The figure shows three views and two pictorial views of one solid part (mm, origin at its lowest corner). Answer the questions. A direction names the side the tool comes from. Coordinates: 2 decimals unless noted, no trailing zeros. Loops run counter-clockwise (first coordinate to the right, second up) from the corner with the lowest first, then second, coordinate; pieces in that order, holes last. Notation, with made-up numbers: M 53,39 L 86,39 A34 cw 86,71 Z; hole C -26,82.5 d5. An arc over 180 degrees is marked long. Return JSON: item names as keys, results as strings. Group by question number.
1. Given P1, Ø2, axis at x = 37, y = 4, coming from the -Z side, flat-ended and moving along its own axis, determine where the tip first touches the part or whether it passes through.
2. Straight lines are drawn through the part: L1, parallel to X at y = 3.15, z = 11; L2, parallel to X at y = 4.6, z = 5; L3, parallel to Z at x = 25, y = 1.6. For each, find the intervals that lie inside material, in ascending order. Write a range as from..to.
3. Which of the six approach directions +Z, -Z, +X, -X, +Y, -Y give full straight-line access (tool end or side, diameter ignored) to the marked faces 1 and 2?
4. Section C-C (y = 4.2) is taken. Write down the section's boundary in (x, z).
5. Section D-D (x = 10.75) is taken. Write down the section's boundary in (y, z), then the cut area to 3 significant figures.
6. Section A-A (x = 24) is taken. Write down the section's boundary in (y, z), then the cut area to 3 significant figures.
7. The mould has two halves that part along X. Classify the marked faces 3, 4 and 5: pulls with the +X half, pulls with the -X half, needs draft (parallel to the pull), parting line crosses it, or undercut.
8. Section B-B (z = 11) is taken. Write down the section's boundary in (x, y), then the cut area to 3 significant figures.
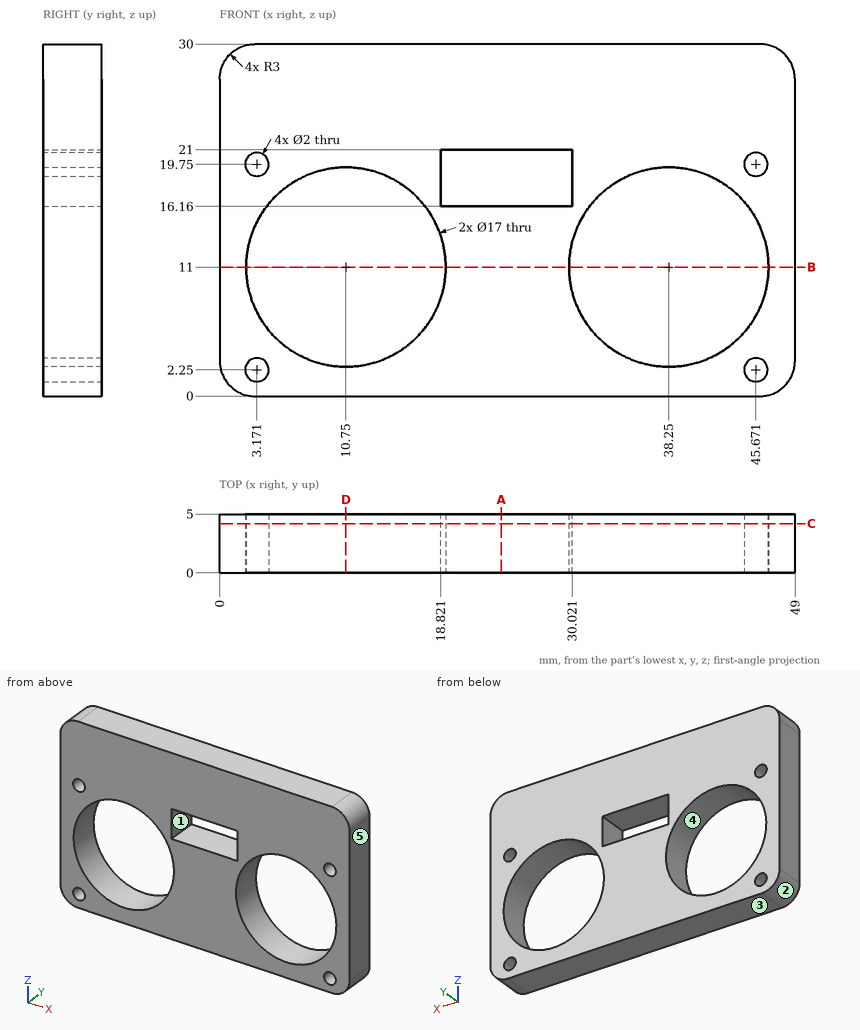
Worked out:
{
 "1": {"P1": "z = 0"},
 "2": {"L1": "0..2.25, 19.25..29.75, 46.75..49", "L2": "0..4.73, 16.77..32.23, 44.27..49", "L3": "0..16.16, 21..30"},
 "3": {"face 1": "+Y, -Y", "face 2": "-Z, -X, +Y, -Y"},
 "4": {"outline": "M 0,3 A3 ccw 3,0 L 46,0 A3 ccw 49,3 L 49,27 A3 ccw 46,30 L 3,30 A3 ccw 0,27 Z; hole C 3.17,2.25 d2; hole C 3.17,19.75 d2; hole C 10.75,11 d17; hole M 18.82,16.16 L 30.02,16.16 L 30.02,21 L 18.82,21 Z; hole C 38.25,11 d17; hole C 45.67,2.25 d2; hole C 45.67,19.75 d2"},
 "5": {"outline": "M 0,0 L 5,0 L 5,2.5 L 0,2.5 Z; M 0,19.5 L 5,19.5 L 5,30 L 0,30 Z", "area": "65.0 mm^2"},
 "6": {"outline": "M 0,0 L 5,0 L 5,16.16 L 0,16.16 Z; M 0,21 L 5,21 L 5,30 L 0,30 Z", "area": "126 mm^2"},
 "7": {"face 3": "needs draft", "face 4": "undercut", "face 5": "pulls with the +X half"},
 "8": {"outline": "M 0,0 L 2.25,0 L 2.25,5 L 0,5 Z; M 19.25,0 L 29.75,0 L 29.75,5 L 19.25,5 Z; M 46.75,0 L 49,0 L 49,5 L 46.75,5 Z", "area": "75.0 mm^2"}
}
